Print and shaded views of the part. All mm, measured from the part's lowest x, y and z. A direction names the side the tool comes from. Give positions to 0.01 mm unless a question says otherwise; leave off trailing zeros. Write each loop counter-clockwise with the first axis right and the second up, starting at its lowest first coordinate (ties: lowest second). Pieces come first, ordered by that corner, then holes. Notation, with made-up numbers: M 53.25,39 L 100.25,39 A11 cw 100.25,56 Z; hole C 41.25,-6.5 d1. An arc over 180 degrees is marked long. One line per question, with ' | ' between items. Start each with the question number.
1. Cut at A-A, the plane x = 2.65. Write the cut outline in (y, z).
2. Which spindle directions (+Z, -Z, +X, -X, +Y, -Y) get a long thin tool onto all of the face, cutting with end or side? Do the marked faces 1 and 2. Say none if no direction does.
3. Wall check: L1, parallel to Y at x = 3.8, z = 5.4; L2, parallel to Z at x = 2.65, y = 2.95; L3, parallel to Z at x = 1.6, y = 0.75 (1 decimal). Give the ranges that are in metal, low to high.
4. Cut at C-C, the plane y = 3.7. Write the cut outline in (x, z), then the cut area to 3 significant figures.
5. Cut at B-B, the plane z = 2.9. Write the cut outline in (x, y).
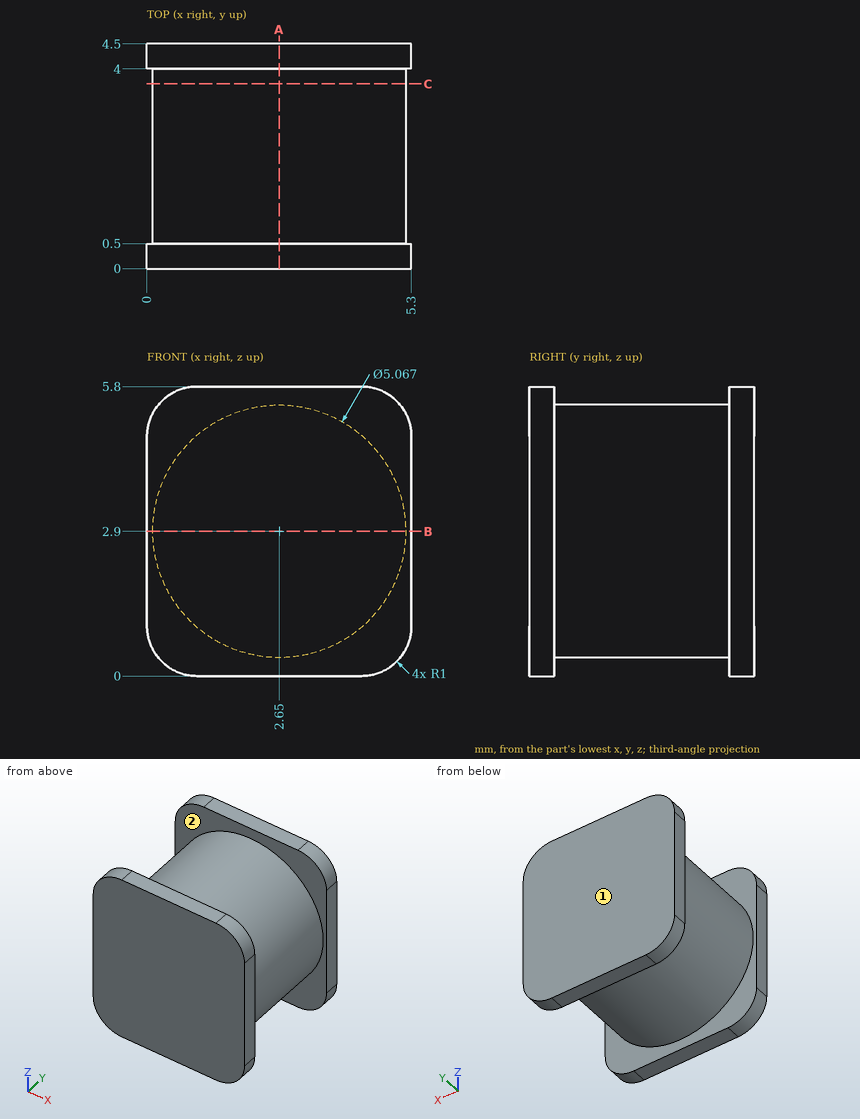
Here are the results:
1) outline: M 0,0 L 0.5,0 L 0.5,0.37 L 4,0.37 L 4,0 L 4.5,0 L 4.5,5.8 L 4,5.8 L 4,5.43 L 0.5,5.43 L 0.5,5.8 L 0,5.8 Z
2) face 1: +Z, -Z, +X, -X, +Y | face 2: none
3) L1: 0 to 0.5, 4 to 4.5 | L2: 0.37 to 5.43 | L3: 0.6 to 5.2
4) outline: C 2.65,2.9 d5.07 | area: 20.2 mm^2
5) outline: M 0,0 L 5.3,0 L 5.3,0.5 L 5.18,0.5 L 5.18,4 L 5.3,4 L 5.3,4.5 L 0,4.5 L 0,4 L 0.12,4 L 0.12,0.5 L 0,0.5 Z
